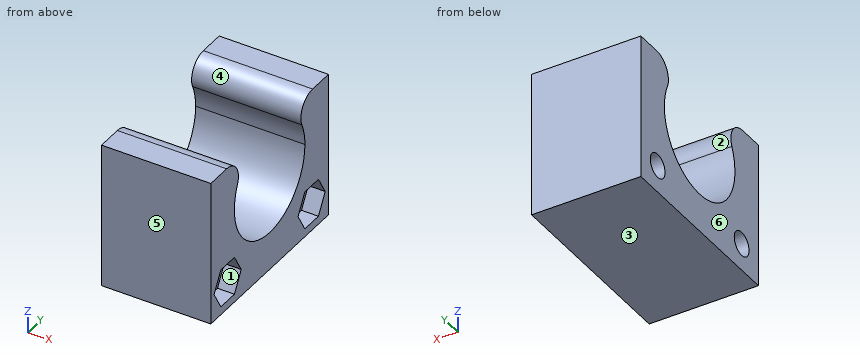
```python
from build123d import *

# Parameters (mm, degrees)
F0_W     = 35
F0_H     = 35
F1_DEPTH = 20
F3_DEPTH = 51.098119
F4_R     = 3.5
F6_DEPTH = 3.1
F8_D     = 4.4


with BuildPart() as f1:
    # F0 (on Right) → F1 (new body)
    with BuildSketch(Plane.YZ):
        Rectangle(F0_W, F0_H)
    extrude(amount=F1_DEPTH)

    # F2 (on face) → F3 (cut)
    with BuildSketch(Plane.YZ.offset(20)):
        with BuildLine():
            ThreePointArc((-5.10385, 9.176094), (-5.322573, -9.050979), (10.5, 0))
            ThreePointArc((10.5, 0), (9.050979, 5.322573), (5.10385, 9.176094))
            ThreePointArc((5.10385, 9.176094), (0, 10.5), (-5.10385, 9.176094))
        make_face()
        with BuildLine():
            ThreePointArc((-5.10385, 9.176094), (0, 10.5), (5.10385, 9.176094))
            Line((5.10385, 9.176094), (17.5, 9.176094))
            Line((17.5, 9.176094), (17.5, 17.5))
            Line((17.5, 17.5), (-17.5, 17.5))
            Line((-17.5, 17.5), (-17.5, 9.176094))
            Line((-17.5, 9.176094), (-5.10385, 9.176094))
        make_face()
    extrude(amount=-F3_DEPTH, mode=Mode.SUBTRACT)

    # F4
    f4_edges = [f1.edges().sort_by_distance(p)[0] for p in [
        (10, 5.10385, 9.176094),
        (10, -5.10385, 9.176094),
    ]]
    fillet(f4_edges, radius=F4_R)

    # F5 (on face) → F6 (cut)
    with BuildSketch(Plane.YZ.offset(20)):
        Polygon((10.479274, -16), (14.520726, -16), (16.541452, -12.5), (14.520726, -9), (10.479274, -9), (8.458548, -12.5), align=None)
        Polygon((-8.458548, -12.5), (-10.479274, -9), (-14.520726, -9), (-16.541452, -12.5), (-14.520726, -16), (-10.479274, -16), align=None)
    extrude(amount=-F6_DEPTH, mode=Mode.SUBTRACT)

    # F8 (through all)
    with Locations(Plane(origin=(0, 0, 0), x_dir=(0, -1, 0), z_dir=(-1, 0, 0))):
        with Locations((-12.5, -12.5), (12.5, -12.5)):
            Hole(F8_D / 2)


solid = f1.part
```
Model file for the job. Use its own axes, mm. Face numbers are marked on the shaded views. A direction names the side the tool comes from. Coordinates: 2 decimals unless noted, no trailing zeros. Order: outer loops, then holes, each group sorted by start corner. A loop starts at its lowest first (then second) coordinate and runs counter-clockwise, first axis right, second up. Notation, with made-up numbers: (-2, -23) -> (51, -23) arc R19 cw to (51, -12) -> close; hole circle Ø1 at (-27.75, 42.25). An arc over 180 degrees is marked (long way). Return JSON: item names as keys, results as strings.
Item 1: Slice it at D-D (y = 0). Write the cut outline in (x, z), then the cut area to 3 significant figures.
Model answer:
{"outline": "(0, -17.5) -> (20, -17.5) -> (20, -10.5) -> (0, -10.5) -> close", "area": "140 mm²"}
Item 2: 3-axis set-ups, long thin cutter, end or side, ignore diameter. For the marked faces 1, 2 and 3: which of +Z, -Z, +X, -X, +Y, -Y reach the whole face in a straight line?
Model answer:
{"face 1": "+X", "face 2": "+X, -X", "face 3": "-Z, +X, -X, +Y, -Y"}
Item 3: Slice it at A-A (y = 12). Write the cut outline in (x, z), then the cut area to 3 significant figures.
Model answer:
{"outline": "(0, -17.5) -> (20, -17.5) -> (20, -16) -> (16.9, -16) -> (16.9, -14.64) -> (0, -14.64) -> close; (0, -10.36) -> (16.9, -10.36) -> (16.9, -9) -> (20, -9) -> (20, 9.08) -> (0, 9.08) -> close", "area": "438 mm²"}
Item 4: Mould opens along Y. For the marked faces 4, 5 and 6 say: pulls with the +Y half, pulls with the -Y half, needs draft (parallel to the pull), parting line crosses it, or undercut.
Model answer:
{"face 4": "undercut", "face 5": "pulls with the -Y half", "face 6": "needs draft"}
Item 5: Slice it at B-B (z = 0.75). Write the cut outline in (x, y), then the cut area to 3 significant figures.
Model answer:
{"outline": "(0, -17.5) -> (20, -17.5) -> (20, -10.47) -> (0, -10.47) -> close; (0, 10.47) -> (20, 10.47) -> (20, 17.5) -> (0, 17.5) -> close", "area": "281 mm²"}
Item 6: Wall check: line 1 along Y through (x, z) = (5.5, -14.5); line 2 along Y through (x, z) = (7.5, 0); line 3 along Y through (x, z) = (18.25, -14.5). Give the ranges that are in metal, low to high. Write a range as from..to.
Model answer:
{"line 1": "y = -17.5..-13.42, -11.58..11.58, 13.42..17.5", "line 2": "y = -17.5..-10.5, 10.5..17.5", "line 3": "y = -17.5..-15.39, -9.61..9.61, 15.39..17.5"}
Item 7: Pin check, flat tips, straight feed: P1, Ø6, axis at x = 15.5, y = -8, coming from the +Z side; P2, Ø4, axis at x = 3, y = -10.5, coming from the +Z side; P3, Ø7.5, axis at y = -11.5, z = -11.5, coming from the +X side; P4, Ø5.5, axis at y = -12.5, z = -12.5, coming from the +X side. Stop position of each tip, or through.
Model answer:
{"P1": "stops at z = 8.68", "P2": "stops at z = 9.16", "P3": "stops at x = 20", "P4": "stops at x = 16.9"}
Item 8: Slice it at C-C (x = 18.5). Write the cut outline in (y, z), then the cut area to 3 significant figures.
Model answer:
{"outline": "(-17.5, -17.5) -> (17.5, -17.5) -> (17.5, 9.18) -> (12.8, 9.18) arc R3.5 ccw to (9.6, 4.26) arc R10.5 cw to (10.5, 0) arc R10.5 cw (long way) to (-9.6, 4.26) arc R3.5 ccw to (-12.8, 9.18) -> (-17.5, 9.18) -> close; hole (-16.54, -12.5) -> (-14.52, -16) -> (-10.48, -16) -> (-8.46, -12.5) -> (-10.48, -9) -> (-14.52, -9) -> close; hole (8.46, -12.5) -> (10.48, -16) -> (14.52, -16) -> (16.54, -12.5) -> (14.52, -9) -> (10.48, -9) -> close", "area": "492 mm²"}
